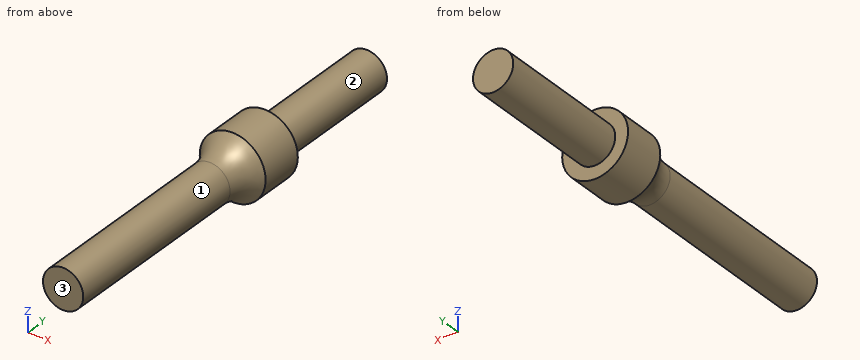
```python
from build123d import *

# Parameters (mm, degrees)
FILLET_1_R      = 3
SKETCH_3_R      = 1.375
EXTRUDE_2_DEPTH = 2.5


with BuildPart() as part:
    # Эскиз1 → Повернуть1 (revolve)
    with BuildSketch(Plane(origin=(0, 0, -25.3000002), x_dir=(-1, 0, 0), z_dir=(0, 0, -1)), mode=Mode.PRIVATE) as revolve_1_sk:
        Polygon((-39.00000074, -6.09116098), (-39.00000074, 19.69999898), (-40.37500074, 19.69999898), (-40.37500074, 12.69999898), (-41.25000074, 12.69999898), (-41.25000074, 9.69999898), (-40.37500074, 9.69999898), (-40.37500074, -6.09116098), align=None)
    revolve(revolve_1_sk.sketch.rotate(Axis((39.00000074, -6.09116098, -25.3000002), (0, 1, 0)), 90), axis=Axis((39.00000074, -6.09116098, -25.3000002), (0, 1, 0)))

    # Скругление1
    # the kernel refuses this fillet: 3 mm, written as the material it adds along each edge
    with BuildSketch(Plane(origin=(39.00000074, 9.69999898, -25.3000002), x_dir=(0, 0, -1), z_dir=(1, 0, 0))) as fillet_1_piece_1:
        with BuildLine():
            CenterArc((4.375, -2.117634293), FILLET_1_R, 135.099472039, 44.900527961)
            Line((1.375, -2.117634293), (1.315, -2.117634293))
            Line((1.315, -2.117634293), (1.315, 0))
            Line((1.315, 0), (1.375, 0.06))
            ThreePointArc((1.375, 0.06), (1.8125, 0.06), (2.2075, 0.042352686))
            Line((2.2075, 0.042352686), (2.25, 0))
        make_face()
    revolve(axis=Axis((39.00000074, 9.69999898, -25.3000002), (0, 1, 0)))

    # Эскиз3 → Бобышка-Вытянуть2 (add)
    with BuildSketch(Plane(origin=(0, 19.69999898, 0), x_dir=(1, 0, 0), z_dir=(0, 1, 0))):
        with Locations(Location((39.00000074, 25.3000002, 0), (0, 0, 90))):
            Circle(SKETCH_3_R)
    extrude(amount=EXTRUDE_2_DEPTH)


solid = part.part
```
Check sheet for the modelled part. Datum: model origin and axes. Units: mm. Face numbers are marked on the shaded views. A direction names the side the tool comes from. Round coordinates to 2 decimals unless told otherwise and drop trailing zeros. Write each loop counter-clockwise with the first axis right and the second up, starting at its lowest first coordinate (ties: lowest second). Pieces come first, ordered by that corner, then holes. Notation, with made-up numbers: (24, -29.5) -> (66, -29.5) arc R23 cw to (66, -7.5) -> close; hole circle Ø11 at (9, 60). An arc over 180 degrees is marked (long way). One line per question, with ' | ' between items. Start each with the question number.
1. Depth check by flat-ended pin: pin 1 (2 mm diameter, centred on x = 38.5, z = -27, fed in from -Y); pin 2 (1 mm diameter, centred on x = 37.5, y = 1.5, fed in from +Z); pin 3 (1.5 mm diameter, centred on y = 5, z = -26.5, fed in from +X). Enter the tip coordinate at first touch or a pass-through.
2. Scan lines: line 1 along X through (y, z) = (-2.25, -26.45); line 2 along Z through (x, y) = (39.6, 13.5); line 3 along Z through (x, y) = (39.5, 19). Record each from-to range of solid material in increasing order. Write a range as from..to.
3. Sectioned sample at B-B, the plane y = 11.5. Record the cut outline in (x, z), then the cut area to 3 significant figures.
4. Set-up check for the marked faces 1, 2 and 3: record each of +Z, -Z, +X, -X, +Y, -Y from which the full face is reachable in a straight line by a thin tool's end or side.
5. Sectioned sample at A-A, the plane y = 0.25. Record the cut outline in (x, z) (3 decimals), then the cut area to 3 significant figures.
Taken from the geometry:
1) pin 1: stops at y = -6.09 | pin 2: stops at z = -24.36 | pin 3: stops at x = 40.3
2) line 1: x = 38.25..39.75 | line 2: z = -26.54..-24.06 | line 3: z = -26.58..-24.02
3) outline: circle Ø4.5 at (39, -25.3) | area: 15.9 mm^2
4) face 1: -Y | face 2: +Y | face 3: +Z, -Z, +X, -X, -Y
5) outline: circle Ø2.75 at (39, -25.3) | area: 5.94 mm^2
